Read the model definition and answer for the solid it produces. Units are mm, in the model's axes. A direction names the side the tool comes from. Coordinates: 2 decimals unless noted, no trailing zeros. Order: outer loops, then holes, each group sorted by start corner. A loop starts at its lowest first (then second) coordinate and runs counter-clockwise, first axis right, second up. Notation, with made-up numbers: M -22,39 L -17,39 A23 cw -17,74 Z; hole C 50,30.5 d3. An arc over 180 degrees is marked long. One line per question, with ' | ' between items. Start each with the question number.
1) Find section A-A, the plane y = 0. Write down the section's boundary in (x, z).
2) Find section D-D, the plane z = 15. Write down the section's boundary in (x, y), plus the area to 3 significant figures.
3) Find section C-C, the plane x = 0. Write down the section's boundary in (y, z), plus the area to 3 significant figures.
4) Given P1, Ø4, axis at x = -1.5, y = 0, coming from the -Z side; P2, Ø10, axis at x = -12.5, z = 1, coming from the +Y side; P3, Ø10, axis at y = 6, z = 5.5, coming from the -X side, each flat-ended and moving along its own axis, determine where each tip first touches the part or whether it passes through.
5) The mould has two halves that part along Y. Classify faces 3 (the face through (0, 0, 18.5)), 4 (the face through (1.63, 0, 6)), 5 (the face through (15.24, -6.32, 7.37)): +Y half, -Y half, draft (parallel to the pull), parting line (faces both ways), or undercut.
6) Find section B-B, the plane z = 9.5. Write down the section's boundary in (x, y), plus the area to 3 significant figures.
7) Consider probe 1 along Y at (x, z) = (0, 1.55); probe 2 along Y at (x, z) = (0, 7.25); probe 3 along Z at (x, y) = (-11.5, 9). Determine where each line is inside the solid, lowest interval first.
8) A tool of negligible diameter and unlimited length cuts with its end or side. For faces 1 (the face through (0, -7, -1.5)), 2 (the face through (0, 0, 10)), from which of +Z, -Z, +X, -X, +Y, -Y can it reach the whole face along a straight path? Write none if from no direction.
from build123d import *

# Parameters (mm, degrees)
CYLINDER022_R     = 6
CYLINDER022_DEPTH = 4.5
PAD105_DEPTH      = 7
CYLINDER007_R     = 16.5
CYLINDER007_DEPTH = 20
FILLET013_R       = 2


with BuildPart() as obj1:
    # Cylinder022 → Cylinder022 (new body)
    with BuildSketch(Plane.XY.offset(-1.5)):
        Circle(CYLINDER022_R)
    extrude(amount=CYLINDER022_DEPTH)


with BuildPart() as obj2:
    # Sketch082 → Pad105 (new body)
    with BuildSketch(Plane.XY):
        with BuildLine():
            Line((1.630229, 2.85), (1.630229, -2.85))
            ThreePointArc((1.630229, 2.85), (-3.283313, 0), (1.630229, -2.85))
        make_face()
    extrude(amount=PAD105_DEPTH)


with BuildPart() as obj2_1:
    # Body018 placement: moved
    add(obj2.part.moved(Location((0, 0, 3))))


with BuildPart() as obj3:
    # Cylinder007 → Cylinder007 (new body)
    with BuildSketch(Plane.XY.offset(-1.5)):
        Circle(CYLINDER007_R)
    extrude(amount=CYLINDER007_DEPTH)

    # Cut018: cut obj2
    add(obj2_1.part, mode=Mode.SUBTRACT)

    # Cut024: cut obj1
    add(obj1.part, mode=Mode.SUBTRACT)

    # Fillet013
    fillet013_edges = [obj3.edges().sort_by_distance(p)[0] for p in [
        (-16.5, 0, 18.5),
    ]]
    fillet(fillet013_edges, radius=FILLET013_R)


solid = obj3.part
Report:
1) outline: M -16.5,-1.5 L -6,-1.5 L -6,3 L -3.28,3 L -3.28,10 L 1.63,10 L 1.63,3 L 6,3 L 6,-1.5 L 16.5,-1.5 L 16.5,16.5 A2 ccw 14.5,18.5 L -14.5,18.5 A2 ccw -16.5,16.5 Z
2) outline: C 0,0 d33 | area: 855 mm^2
3) outline: M -16.5,-1.5 L -6,-1.5 L -6,3 L -3.28,3 L -3.28,10 L 3.28,10 L 3.28,3 L 6,3 L 6,-1.5 L 16.5,-1.5 L 16.5,16.5 A2 ccw 14.5,18.5 L -14.5,18.5 A2 ccw -16.5,16.5 Z | area: 558 mm^2
4) P1: stops at z = 3 | P2: stops at y = 14.7 | P3: stops at x = -16.47
5) face 3: draft | face 4: undercut | face 5: parting line
6) outline: C 0,0 d33; hole M 1.63,-2.85 L 1.63,2.85 A3.28 ccw long Z | area: 828 mm^2
7) probe 1: y = -16.5 to -6, 6 to 16.5 | probe 2: y = -16.5 to -3.28, 3.28 to 16.5 | probe 3: z = -1.5 to 18.5
8) face 1: -Z, +X, -X, +Y, -Y | face 2: -Z
